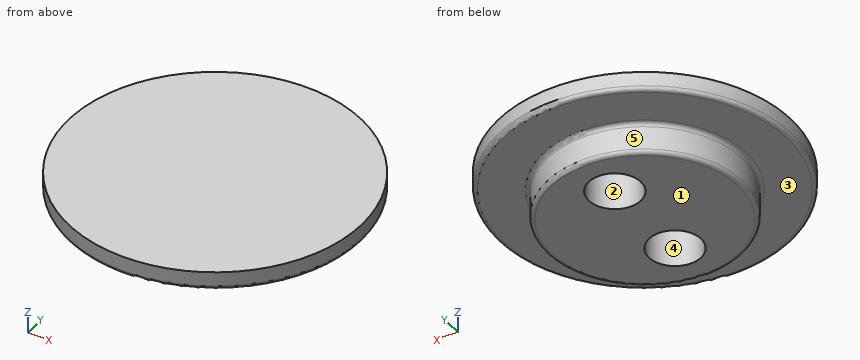
from build123d import *

# Parameters (mm, degrees)
SKETCH1_R           = 18.65
BOSS_EXTRUDE1_DEPTH = 2.3495
SKETCH4_R           = 12.446
BOSS_EXTRUDE2_DEPTH = 4.0005
SKETCH5_R           = 3.3275
CUT_EXTRUDE1_DEPTH  = 5.85
FILLET1_R           = 0.508


with BuildPart() as part:
    # Sketch1 → Boss-Extrude1 (new body)
    with BuildSketch(Plane.XY):
        with Locations((-43, 22.86)):
            Circle(SKETCH1_R)
    extrude(amount=-BOSS_EXTRUDE1_DEPTH)

    # Sketch4 → Boss-Extrude2 (add)
    with BuildSketch(Plane(origin=(0, 0, -2.3495), x_dir=(-1, 0, 0), z_dir=(0, 0, -1))):
        with Locations(Location((43, 22.86, 0), (0, 0, 180))):
            Circle(SKETCH4_R)
    extrude(amount=BOSS_EXTRUDE2_DEPTH)

    # Sketch5 → Cut-Extrude1 (cut)
    with BuildSketch(Plane(origin=(0, 0, -6.35), x_dir=(-1, 0, 0), z_dir=(0, 0, -1))):
        with Locations((43, 29.083)):
            Circle(SKETCH5_R)
        with Locations(Location((43, 16.637, 0), (0, 0, 180))):
            Circle(SKETCH5_R)
    extrude(amount=-CUT_EXTRUDE1_DEPTH, mode=Mode.SUBTRACT)

    # Fillet1
    fillet1_edges = [part.edges().sort_by_distance(p)[0] for p in [
        (-61.65, 22.86, -2.3495),
        (-55.446, 22.86, -2.3495),
        (-55.446, 22.86, -6.35),
    ]]
    fillet(fillet1_edges, radius=FILLET1_R)


solid = part.part
Geometry check sheet. Reference: the model listing, model coordinates, mm. Face numbers are marked on the shaded views. A direction names the side the tool comes from. Give positions to 0.01 mm unless a question says otherwise; leave off trailing zeros. Loops run counter-clockwise (first coordinate to the right, second up) from the corner with the lowest first, then second, coordinate; pieces in that order, holes last. Notation, with made-up numbers: (-17.75, 69) -> (24.25, 69) arc R16 cw to (24.25, 77) -> close; hole circle Ø5 at (52.5, -27.5). An arc over 180 degrees is marked (long way). Answer in a Markdown table with one row per item. Add a question column.
1) Set-up check for the marked faces 1 and 2: record each of +Z, -Z, +X, -X, +Y, -Y from which the full face is reachable in a straight line by a thin tool's end or side.
2) Draft check along Y on the marked faces 3, 4 and 5. Enter one of: pulls with the +Y half, pulls with the -Y half, needs draft (parallel to the pull), parting line crosses it, or undercut.
3) Gauge pin test, flat ends, axial feed: P1, Ø5.5, axis at x = -43, y = 16.637, coming from the -Z side; P2, Ø3, axis at x = -31, z = -3, coming from the -Y side. Record the tip position at first contact, or that the pin passes through.
4) Material ranges on probe 1 along Y at (x, z) = (-43, -4.8); probe 2 along Y at (x, z) = (-40.5, -5.75); probe 3 along Z at (x, y) = (-58.5, 18), recorded low to high. Write a range as from..to.
5) Cross-section at B-B on y = 22.86. Record the boundary of the cut face in (x, z).
6) Cross-section at A-A on x = -43. Record the boundary of the cut face in (y, z).
Outcome:
| question | item | result |
|---|---|---|
| 1 | face 1 | -Z, +X, -X, +Y, -Y |
| 1 | face 2 | -Z |
| 2 | face 3 | needs draft |
| 2 | face 4 | undercut |
| 2 | face 5 | parting line crosses it |
| 3 | P1 | stops at z = -0.5 |
| 3 | P2 | stops at y = 7.74 |
| 4 | probe 1 | y = 10.41..13.31, 19.96..25.76, 32.41..35.31 |
| 4 | probe 2 | y = 10.67..14.44, 18.83..26.89, 31.28..35.05 |
| 4 | probe 3 | z = -2.35..0 |
| 5 | outline | (-61.65, -1.84) arc R0.51 ccw to (-61.14, -2.35) -> (-55.95, -2.35) arc R0.51 cw to (-55.45, -2.86) -> (-55.45, -5.84) arc R0.51 ccw to (-54.94, -6.35) -> (-31.06, -6.35) arc R0.51 ccw to (-30.55, -5.84) -> (-30.55, -2.86) arc R0.51 cw to (-30.05, -2.35) -> (-24.86, -2.35) arc R0.51 ccw to (-24.35, -1.84) -> (-24.35, 0) -> (-61.65, 0) -> close |
| 6 | outline | (4.21, -1.84) arc R0.51 ccw to (4.72, -2.35) -> (9.91, -2.35) arc R0.51 cw to (10.41, -2.86) -> (10.41, -5.84) arc R0.51 ccw to (10.92, -6.35) -> (13.31, -6.35) -> (13.31, -0.5) -> (19.96, -0.5) -> (19.96, -6.35) -> (25.76, -6.35) -> (25.76, -0.5) -> (32.41, -0.5) -> (32.41, -6.35) -> (34.8, -6.35) arc R0.51 ccw to (35.31, -5.84) -> (35.31, -2.86) arc R0.51 cw to (35.81, -2.35) -> (41, -2.35) arc R0.51 ccw to (41.51, -1.84) -> (41.51, 0) -> (4.21, 0) -> close |
